Source: three-view drawing plus pictorial views. Frame: mm from the lowest corner of the part. A direction names the side the tool comes from. Round coordinates to 2 decimals unless told otherwise and drop trailing zeros. Loops run counter-clockwise (first coordinate to the right, second up) from the corner with the lowest first, then second, coordinate; pieces in that order, holes last. Notation, with made-up numbers: (34.5, 81) -> (83.5, 81) arc R12 cw to (83.5, 95) -> close; hole circle Ø1 at (37.25, 69). An arc over 180 degrees is marked (long way). Answer in a Markdown table with one row per item.
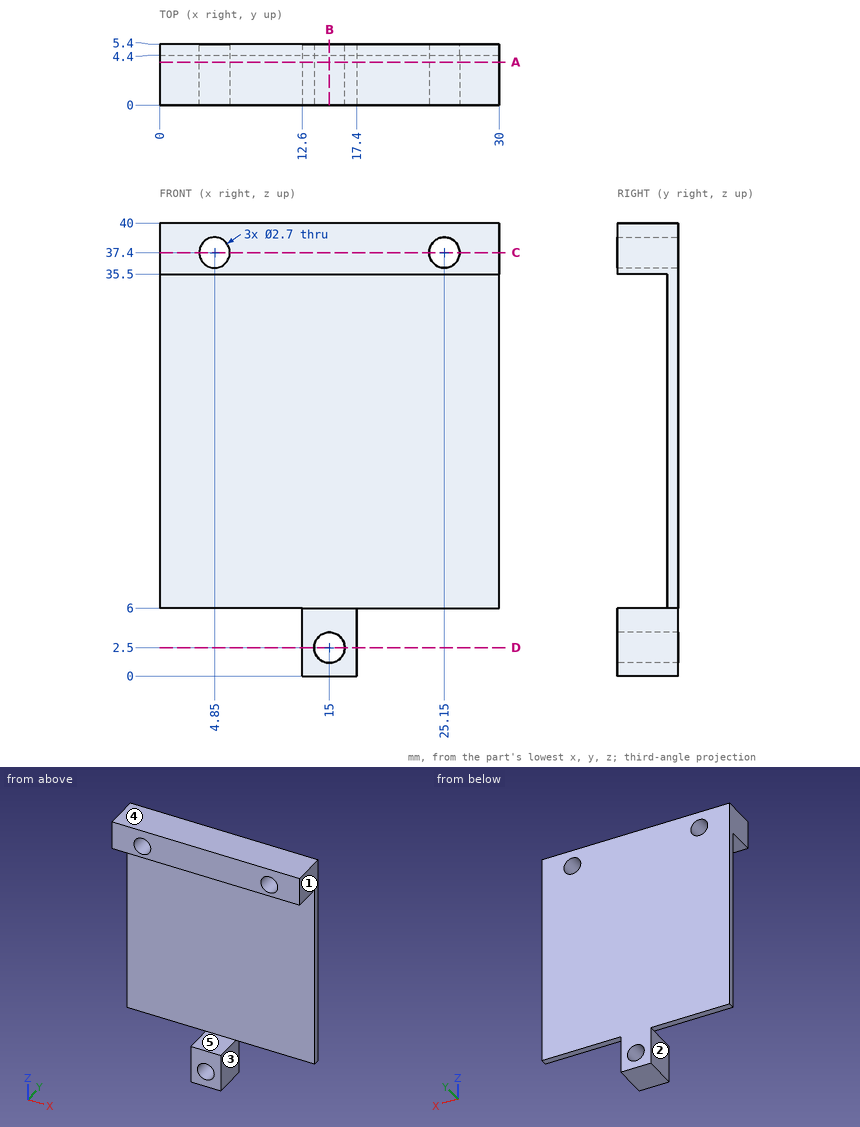
Item 1: Reachability of the marked faces 1 and 2 from +Z, -Z, +X, -X, +Y, -Y: full face, straight path, thin tool, end or side. Return the list, or none.
Answer:
| item | result |
|---|---|
| face 1 | +Z, -Z, +X, +Y, -Y |
| face 2 | -Z, -X, +Y, -Y |
Item 2: Cut plane A-A (y = 3.8). Output: boundary loops of the cut face in (x, z).
Answer:
| item | result |
|---|---|
| outline | (0, 35.5) -> (30, 35.5) -> (30, 40) -> (0, 40) -> close; (12.6, 0) -> (17.4, 0) -> (17.4, 6) -> (12.6, 6) -> close; hole circle Ø2.7 at (4.85, 37.4); hole circle Ø2.7 at (15, 2.5); hole circle Ø2.7 at (25.15, 37.4) |
Item 3: Cut plane B-B (x = 15). Output: boundary loops of the cut face in (y, z).
Answer:
| item | result |
|---|---|
| outline | (0, 0) -> (5.4, 0) -> (5.4, 1.15) -> (0, 1.15) -> close; (0, 3.85) -> (5.4, 3.85) -> (5.4, 40) -> (0, 40) -> (0, 35.5) -> (4.4, 35.5) -> (4.4, 6) -> (0, 6) -> close |
Item 4: Pin query (flat end, axial travel): pin 1 Ø3 at (x, z) = (14, 25.5) entering from -Y; pin 2 Ø1.1 at (x, y) = (25.5, 4.5) entering from -Z; pin 3 Ø1.6 at (y, z) = (3.5, 4.5) entering from -X. Return the tip coordinate at first contact, or that it passes through.
Answer:
| item | result |
|---|---|
| pin 1 | stops at y = 4.4 |
| pin 2 | stops at z = 6 |
| pin 3 | stops at x = 12.6 |
Item 5: Cut plane D-D (z = 2.5). Output: boundary loops of the cut face in (x, y).
Answer:
| item | result |
|---|---|
| outline | (12.6, 0) -> (13.65, 0) -> (13.65, 5.4) -> (12.6, 5.4) -> close; (16.35, 0) -> (17.4, 0) -> (17.4, 5.4) -> (16.35, 5.4) -> close |
Item 6: Line query: probe 1 along Z at (x, y) = (15, 2.35); probe 2 along Z at (x, y) = (13.5, 1.05); probe 3 along Z at (x, y) = (25.15, 3.55). Output: solid intervals per line, ascending. Write a range as [from, to].
Answer:
| item | result |
|---|---|
| probe 1 | z = [0, 1.15], [3.85, 6], [35.5, 40] |
| probe 2 | z = [0, 6], [35.5, 40] |
| probe 3 | z = [35.5, 36.05], [38.75, 40] |
Item 7: Draft query along Z for the marked faces 3, 4 and 5. Return one class per face: pulls with the +Z half, pulls with the -Z half, needs draft (parallel to the pull), parting line crosses it, or undercut.
Answer:
| item | result |
|---|---|
| face 3 | needs draft |
| face 4 | pulls with the +Z half |
| face 5 | undercut |
Item 8: Cut plane C-C (z = 37.4). Output: boundary loops of the cut face in (x, y), then the cut area to 3 significant figures.
Answer:
| item | result |
|---|---|
| outline | (0, 0) -> (3.5, 0) -> (3.5, 5.4) -> (0, 5.4) -> close; (6.2, 0) -> (23.8, 0) -> (23.8, 5.4) -> (6.2, 5.4) -> close; (26.5, 0) -> (30, 0) -> (30, 5.4) -> (26.5, 5.4) -> close |
| area | 133 mm² |
